Model file for the job. Use its own axes, mm. A direction names the side the tool comes from. Give positions to 0.01 mm unless a question says otherwise; leave off trailing zeros. Write each loop counter-clockwise with the first axis right and the second up, starting at its lowest first coordinate (ties: lowest second). Pieces come first, ordered by that corner, then holes. Notation, with made-up numbers: M 57,4.5 L 100,4.5 A30 cw 100,31.5 Z; hole C 48.5,49 d9. An arc over 180 degrees is marked long. Answer as a JSON object with one key per item and string values. Group by question number.
Autodesk Inventor part; units mm, degrees
ref_plane "YZ Plane" through (0, 0, 0) normal (1, 0, 0) x (0, 1, 0)
ref_plane "XZ Plane" through (0, 0, 0) normal (0, 1, 0) x (-1, 0, 0)
ref_plane "XY Plane" through (0, 0, 0) normal (0, 0, 1) x (1, 0, 0)
sketch "Sketch1" plane through (0, 0, 0) normal (0, 0, 1) x (1, 0, 0)
  circle A0 centre (0, 0) radius 8.5
  arc A1 (23.5, 0) -> (-23.5, 0) centre (0, 0) ccw
  line L0 (-23.5, 0) -> (-23.5, -50)
  line L1 (-23.5, -50) -> (-15, -58.5)
  line L2 (-15, -58.5) -> (-15, -108.5)
  line L3 (-15, -108.5) -> (15, -108.5)
  line L4 (15, -108.5) -> (15, -58.5)
  line L5 (15, -58.5) -> (23.5, -50)
  line L6 (23.5, -50) -> (23.5, 0)
  line L7 (0, 0) -> (0, -108.5) construction
  dimension "d162" = 17
  dimension "d163" = 15
  dimension "d164" = 50
  dimension "d165" = 45
  dimension "d166" = 50
  dimension "d167" = 30
extrude "Plate5" add sketch "Sketch1" along normal blind 8
properties part number "PNS-073 stretch tear" material "Stainless Steel"
Q1. Wall check: L1, parallel to Y at x = 0, z = 6.75; L2, parallel to Y at x = 1.5, z = 3.25; L3, parallel to X at y = -71, z = 1.5. Give the ranges that are in metal, low to high.
Q2. Slice it at C-C, the plane y = -93. Write the cut outline in (x, z).
Q3. Drop flat-ended pins along their axis: P1, Ø3, axis at x = 15, z = 6.5, coming from the +Y side; P2, Ø10, axis at x = 0, y = 0, coming from the -Z side; P3, Ø1, axis at x = 17.5, z = 2, coming from the -Y side; P4, Ø1, axis at x = 12.5, z = 4.5, coming from the +Y side. Give the stop position or say it passes through.
Q4. Slice it at A-A, the plane x = 0. Write the cut outline in (y, z), then the cut area to 3 significant figures.
Q5. 3-axis set-ups, long thin cutter, end or side, ignore diameter. For faces 1 (the flat face through (15, -84, 4)), 2 (the cylindrical face through (-0.517, 23.494, 3.944)), 3 (the flat face through (-15, -83, 4)): which of +Z, -Z, +X, -X, +Y, -Y reach the whole face in a straight line?
Q6. Slice it at B-B, the plane z = 5. Write the cut outline in (x, y).
Q7. Two-plate mould, pull along Y, no slides. Class faces 4 (the flat face through (0, -108.5, 4)), 5 (the flat face through (-23.5, -25, 4)), 6 (the cylindrical face through (4.57, -7.167, 3.944)): +Y half, -Y half, draft (parallel to the pull), parting line (faces both ways), or undercut.
Q8. Slice it at D-D, the plane x = -5. Write the cut outline in (y, z), then the cut area to 3 significant figures.
Solved:
{
 "1": {"L1": "y = -108.5 to -8.5, 8.5 to 23.5", "L2": "y = -108.5 to -8.37, 8.37 to 23.45", "L3": "x = -15 to 15"},
 "2": {"outline": "M -15,0 L 15,0 L 15,8 L -15,8 Z"},
 "3": {"P1": "stops at y = 19.24", "P2": "passes through", "P3": "stops at y = -56.5", "P4": "stops at y = 20.21"},
 "4": {"outline": "M -108.5,0 L -8.5,0 L -8.5,8 L -108.5,8 Z; M 8.5,0 L 23.5,0 L 23.5,8 L 8.5,8 Z", "area": "920 mm²"},
 "5": {"face 1": "+Z, -Z, +X, -Y", "face 2": "+Z, -Z, +Y", "face 3": "+Z, -Z, -X, -Y"},
 "6": {"outline": "M -23.5,-50 L -15,-58.5 L -15,-108.5 L 15,-108.5 L 15,-58.5 L 23.5,-50 L 23.5,0 A23.5 ccw -23.5,0 Z; hole C 0,0 d17"},
 "7": {"face 4": "-Y half", "face 5": "draft", "face 6": "undercut"},
 "8": {"outline": "M -108.5,0 L -6.87,0 L -6.87,8 L -108.5,8 Z; M 6.87,0 L 22.96,0 L 22.96,8 L 6.87,8 Z", "area": "942 mm²"}
}
